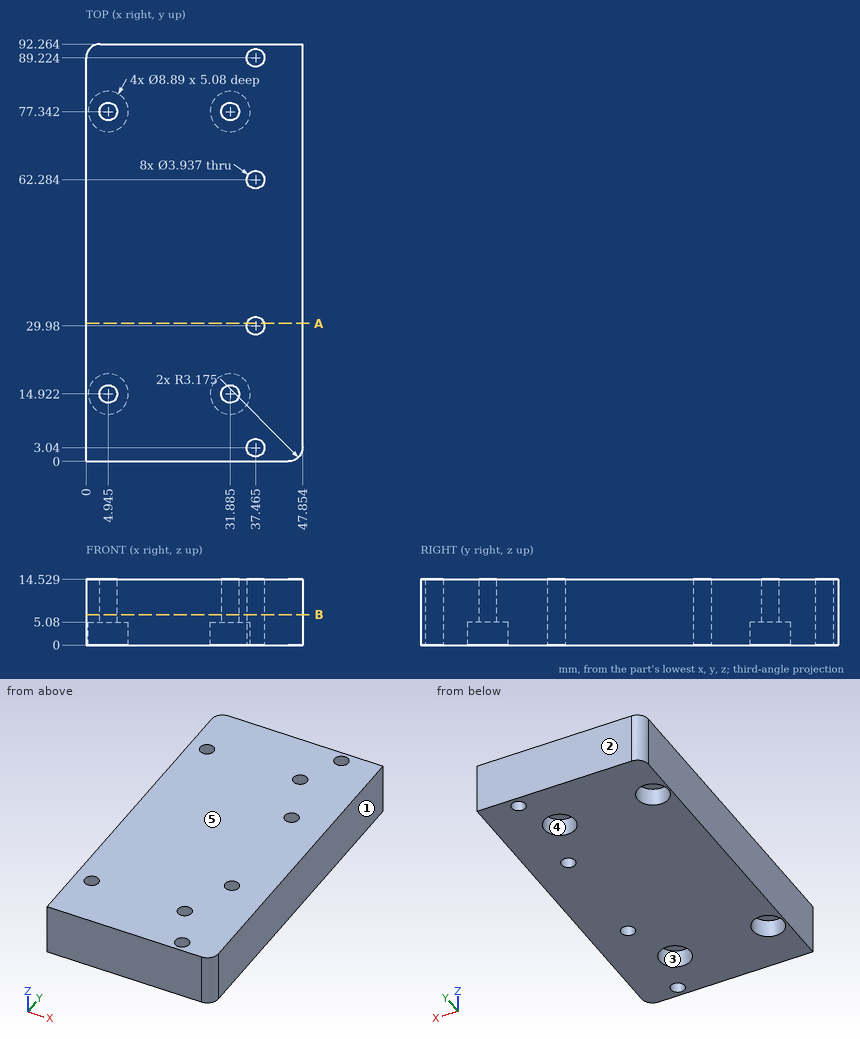
Study the drawing (mm; zero at the part's minimum x, y, z) and answer. A direction names the side the tool comes from. Give positions to 0.01 mm unless a question says otherwise; leave off trailing zeros. Write each loop counter-clockwise with the first axis right and the second up, starting at its lowest first coordinate (ties: lowest second). Pieces come first, ordered by that corner, then holes. Notation, with made-up numbers: (-34, 9.5) - (15, 9.5) arc R27 cw to (15, 29.5) - close; hole circle Ø7 at (-22, -20.5). An arc over 180 degrees is marked (long way). Use a Markdown table: item, result.
1. A tool of negligible diameter and unlimited length cuts with its end or side. For the marked faces 4 and 5, from which of +Z, -Z, +X, -X, +Y, -Y can it reach the whole face along a straight path? Write none if from no direction.
Values follow:
| item | result |
|---|---|
| face 4 | -Z |
| face 5 | +Z, +X, -X, +Y, -Y |
2. Find the intervals of material crossed by probe 1 along Y at (x, z) = (36.5, 9) (1 decimal); probe 2 along Z at (x, y) = (32.5, 79.5); probe 3 along Y at (x, z) = (37, 3) (1 decimal), in increasing order. Write a range as from..to.
Values follow:
| item | result |
|---|---|
| probe 1 | y = 0..1.3, 4.8..28.3, 31.7..60.6, 64..87.5, 90.9..92.3 |
| probe 2 | z = 5.08..14.53 |
| probe 3 | y = 0..1.1, 5..28.1, 31.9..60.4, 64.2..87.3, 91.1..92.3 |
3. Each of these flat-tipped pins is pushed along its axis until it touches: P1, Ø10, axis at x = 34, y = 77.5, coming from the -Z side; P2, Ø5.5, axis at x = 4.94, y = 77.34, coming from the -Z side. Where does it stop, or does it pass through?
Values follow:
| item | result |
|---|---|
| P1 | stops at z = 0 |
| P2 | stops at z = 5.08 |
4. Section A-A on y = 30.5 is taken. Write down the section's boundary in (x, z), plus the area to 3 significant figures.
Values follow:
| item | result |
|---|---|
| outline | (0, 0) - (35.57, 0) - (35.57, 14.53) - (0, 14.53) - close; (39.36, 0) - (47.85, 0) - (47.85, 14.53) - (39.36, 14.53) - close |
| area | 640 mm² |
5. Section B-B on z = 6.75 is taken. Count the separate pieces of the cut face and the enclosed holes in it, plus the area to 3 significant figures.
Values follow:
| item | result |
|---|---|
| separate pieces | 1 |
| enclosed holes | 8 |
| area | 4,310 mm² |
6. For a pull along Y with two mould halves and no side action, classify the marked faces 1, 2 and 3 as released by +Y, released by -Y, zero draft, split by the parting line, or undercut.
Values follow:
| item | result |
|---|---|
| face 1 | zero draft |
| face 2 | released by +Y |
| face 3 | undercut |
